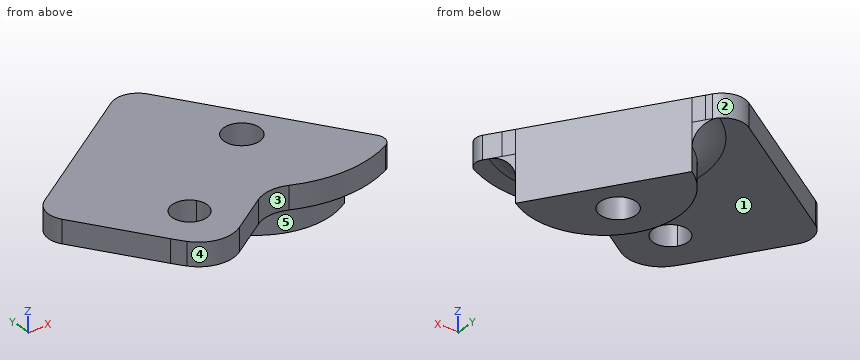
```python
from build123d import *
from build123d.topology import SkipClean

# Parameters (mm, degrees)
EXTRUDE_1_DEPTH     = 2
EXTRUDE_START       = 4
SKETCH_3_R          = 1.55
EXTRUDE_2_DEPTH     = 4
FILLET_1_R          = 2
CUT_EXTRUDE_1_DEPTH = 10
FILLET_2_R          = 2


with BuildPart() as part:
    # 草图2 → 凸台-拉伸1 (new body)
    with BuildSketch(Plane.XY):
        with BuildLine():
            Line((14.564994601, -11.669618141), (7.389813792, -0.829102454))
            Line((7.389813792, -0.829102454), (6.837876806, 0.004783368))
            Line((6.837876806, 0.004783368), (4.07819188, 4.174212479))
            Line((4.07819188, 4.174212479), (3.526254895, 5.008098301))
            Line((3.526254895, 5.008098301), (-3.648925914, 15.848613988))
            Line((-3.648925914, 15.848613988), (-4.2008629, 16.68249981))
            Line((-4.2008629, 16.68249981), (-4.998009984, 17.886857679))
            ThreePointArc((-4.998009984, 17.886857679), (-5.687361464, 18.324420478), (-6.473069172, 18.102316754))
            ThreePointArc((-6.473069172, 18.102316754), (-9.153711125, 14.591132343), (-10.06004351, 10.267613076))
            ThreePointArc((-10.06004351, 10.267613076), (-10.405656258, 8.820717267), (-11.403844954, 7.717732689))
            Line((-11.403844954, 7.717732689), (-14.736003804, 5.512224858))
            ThreePointArc((-14.736003804, 5.512224858), (-15.998358454, 3.706490878), (-15.686779581, 1.525405581))
            ThreePointArc((-15.686779581, 1.525405581), (-15.380816242, 1.008667124), (-15.057770631, 0.502432268))
            Line((-15.057770631, 0.502432268), (-4.019030925, -16.175284173))
            ThreePointArc((-4.019030925, -16.175284173), (-3.679263259, -16.670450943), (-3.323152402, -17.153997481))
            ThreePointArc((-3.323152402, -17.153997481), (-1.437196365, -18.293025266), (0.718231785, -17.83657816))
            Line((0.718231785, -17.83657816), (4.050390635, -15.631070329))
            ThreePointArc((4.050390635, -15.631070329), (5.455716688, -15.143203199), (6.922632961, -15.390412219))
            ThreePointArc((6.922632961, -15.390412219), (11.256585707, -16.245462422), (15.536058254, -15.149847541))
            ThreePointArc((15.536058254, -15.149847541), (16.047506269, -14.513382621), (15.91407867, -13.707861832))
            Line((15.91407867, -13.707861832), (15.116931586, -12.503503963))
            Line((15.116931586, -12.503503963), (14.564994601, -11.669618141))
        make_face()
        with BuildLine():
            ThreePointArc((-1.270469952, 9.628047515), (-3.418495303, 10.065068212), (-3.855516, 7.917042861))
            ThreePointArc((-3.855516, 7.917042861), (-1.707490649, 7.480022164), (-1.270469952, 9.628047515))
        make_face(mode=Mode.SUBTRACT)
        with BuildLine():
            ThreePointArc((7.183223706, -8.76067358), (9.331249057, -9.197694277), (9.768269754, -7.049668926))
            ThreePointArc((9.768269754, -7.049668926), (7.620244403, -6.612648229), (7.183223706, -8.76067358))
        make_face(mode=Mode.SUBTRACT)
        with BuildLine():
            ThreePointArc((-1.947826046, -14.804383569), (0.130908165, -15.227306825), (0.55383142, -13.148572614))
            ThreePointArc((0.55383142, -13.148572614), (-1.524902791, -12.725649358), (-1.947826046, -14.804383569))
        make_face(mode=Mode.SUBTRACT)
        with BuildLine():
            ThreePointArc((-10.484908286, 3.529143828), (-12.563642497, 3.952067083), (-12.986565752, 1.873332872))
            ThreePointArc((-12.986565752, 1.873332872), (-10.907831541, 1.450409617), (-10.484908286, 3.529143828))
        make_face(mode=Mode.SUBTRACT)
    extrude(amount=EXTRUDE_1_DEPTH)

    # 草图3 → 凸台-拉伸2 (add)
    # profile 1 of 2: a face of its own
    with SkipClean():  # the faces are left unmerged after this step: merging them gives an invalid solid
        with BuildSketch(Plane(origin=(0, 0, 0), x_dir=(-1, 0, 0), z_dir=(0, 0, -1)).offset(EXTRUDE_START)):
            with BuildLine():
                ThreePointArc((-3.526254895, 5.008098301), (5.481593353, 6.84076574), (3.648925914, 15.848613988))
                Line((3.648925914, 15.848613988), (-3.526254895, 5.008098301))
            make_face()
            with Locations((2.562992976, 8.772545188)):
                Circle(SKETCH_3_R, mode=Mode.SUBTRACT)
        # profile 2 of 2: a face of its own
        with BuildSketch(Plane(origin=(0, 0, 0), x_dir=(-1, 0, 0), z_dir=(0, 0, -1)).offset(EXTRUDE_START)):
            with BuildLine():
                ThreePointArc((-14.564994601, -11.669618141), (-5.557146353, -9.836950702), (-7.389813792, -0.829102454))
                Line((-7.389813792, -0.829102454), (-14.564994601, -11.669618141))
            make_face()
            with Locations((-8.47574673, -7.905171253)):
                Circle(SKETCH_3_R, mode=Mode.SUBTRACT)
        extrude(amount=-EXTRUDE_2_DEPTH)

    # 圆角1
    # the kernel refuses this fillet: 2 mm, written as the material it adds along each edge
    with BuildSketch(Plane(origin=(10.977404196, -6.249360297, 0), x_dir=(0.5519369853128372, -0.8338858220666526, 0), z_dir=(0.8338858220666526, 0.5519369853128372, 0))) as fillet_1_piece_1:
        with BuildLine():
            CenterArc((6.5 + FILLET_1_R, FILLET_1_R), FILLET_1_R, 180, 90)
            Line((6.5, FILLET_1_R), (6.5, 0))
            Line((6.5, 0), (6.5 + FILLET_1_R, 0))
        make_face()
    revolve(axis=Axis((10.977404196, -6.249360297, 0), (0, 0, -1)), revolution_arc=180)
    with BuildSketch(Plane(origin=(-0.06133551, 10.428356144, 0), x_dir=(0.5519369853122391, -0.8338858220670484, 0), z_dir=(0.8338858220670484, 0.5519369853122391, 0))) as fillet_1_piece_2:
        with BuildLine():
            CenterArc((6.5 + FILLET_1_R, FILLET_1_R), FILLET_1_R, 180, 90)
            Line((6.5, FILLET_1_R), (6.5, 0))
            Line((6.5, 0), (6.5 + FILLET_1_R, 0))
        make_face()
    revolve(axis=Axis((-0.06133551, 10.428356144, 0), (0, 0, -1)), revolution_arc=180)

    # 草图4 → 切除-拉伸1 (cut)
    with BuildSketch(Plane.XY.offset(2)):
        Polygon((5.458034343, 2.089497924), (-9.538400778, -7.836425953), (-26.545257477, 2.73324315), (-0.393587014, 27.879080134), align=None)
    extrude(amount=-CUT_EXTRUDE_1_DEPTH, mode=Mode.SUBTRACT)

    # 圆角2
    # the kernel refuses this fillet: 2 mm, written as the material it takes off along each edge
    with BuildSketch(Plane(origin=(5.458034343, 2.089497924, 7), x_dir=(-0.8338858220669847, -0.5519369853123355, 0), z_dir=(0, 0, -1))) as fillet_2_piece_1:
        with BuildLine():
            CenterArc((FILLET_2_R, -FILLET_2_R), FILLET_2_R, 90, 90)
            Line((0, -FILLET_2_R), (0, 0))
            Line((0, 0), (FILLET_2_R, 0))
        make_face()
    extrude(amount=12, mode=Mode.SUBTRACT)
    with BuildSketch(Plane(origin=(-9.538400778, -7.836425953, 7), x_dir=(0.8338858220669851, 0.5519369853123349, 0), z_dir=(0, 0, -1))) as fillet_2_piece_2:
        with BuildLine():
            CenterArc((FILLET_2_R, FILLET_2_R), FILLET_2_R, 180, 90)
            Line((0, FILLET_2_R), (0, 0))
            Line((0, 0), (FILLET_2_R, 0))
        make_face()
    extrude(amount=12, mode=Mode.SUBTRACT)


solid = part.part
```
The listing builds one solid part. Answer for the finished solid, in the listing's coordinates (mm). Face numbers are marked on the shaded views. A direction names the side the tool comes from. Give positions to 0.01 mm unless a question says otherwise; leave off trailing zeros. Loops run counter-clockwise (first coordinate to the right, second up) from the corner with the lowest first, then second, coordinate; pieces in that order, holes last. Notation, with made-up numbers: (-9.5, 78) - (2.5, 78) arc R26 ccw to (2.5, 116) - close; hole circle Ø2 at (34.25, -14). An arc over 180 degrees is marked (long way). Answer as CSV lines item,"result". Start each with the question number.
Item 1: Find the intervals of material crossed by line 1 (Z direction, x = -2.25, y = -4.75); line 2 (Y direction, x = 7.25, z = 0.75); line 3 (Y direction, x = 13.75, z = -1.25), in increasing order. Write a range as from..to.
Item 2: A cutting plane is placed at A-A on z = 1.5. Count the separate pieces of the cut face and the enclosed holes in it, then the cut area to 3 significant figures.
Item 3: For the marked faces 4 and 5, determine the directions among +Z, -Z, +X, -X, +Y, -Y from which every point of the face is accessible in a straight line to the end or side of a thin tool.
Item 4: Each of these flat-tipped pins is pushed along its axis until it touches: pin 1 (1 mm diameter, centred on x = 5, z = -1, fed in from -Y); pin 2 (6 mm diameter, centred on x = 0, y = -7.5, fed in from -Z); pin 3 (8 mm diameter, centred on x = 0.5, y = -15, fed in from -Z). Where does it stop, or does it pass through?
Item 5: A cutting plane is placed at D-D on z = -2.5. Determine the outline of the cut face in (x, y) (3 decimals).
Item 6: A cutting plane is placed at C-C on x = 1.5. Determine the outline of the cut face in (y, z).
Item 7: A cutting plane is placed at B-B on z = -0.5. Determine the outline of the cut face in (x, y) (3 decimals), then the cut area to 3 significant figures.
Item 8: The mould has two halves that part along X. Classify the marked faces 1, 2 and 3: +X half, -X half, draft (parallel to the pull), parting line (faces both ways), or undercut.
Found:
1,line 1,"z = 0..2"
1,line 2,"y = -15.53..-8.85, -6.96..-0.62"
1,line 3,"y = -12.29..-10.44"
2,separate pieces,"1"
2,enclosed holes,"2"
2,area,"273 mm^2"
3,face 4,"+Z, -Z, -Y"
3,face 5,"-Z"
4,pin 1,"stops at y = -10.47"
4,pin 2,"stops at z = -0.05"
4,pin 3,"stops at z = 0"
5,outline,"(7.39, -0.829) arc R6.5 ccw to (14.565, -11.67) - close; hole circle Ø3.1 at (8.476, -7.905)"
6,outline,"(-17.32, 0) - (-0.53, 0) - (-0.53, 2) - (-17.32, 2) - close"
7,outline,"(7.016, -0.264) arc R7.177 ccw to (14.939, -12.234) - close; hole circle Ø3.1 at (8.476, -7.905)"
7,area,"73.4 mm^2"
8,face 1,"draft"
8,face 2,"parting line"
8,face 3,"undercut"
